CAD build for the part. Positions are in the model's coordinates, mm. Coordinates: 2 decimals unless noted, no trailing zeros. Order: outer loops, then holes, each group sorted by start corner. A loop starts at its lowest first (then second) coordinate and runs counter-clockwise, first axis right, second up.
from build123d import *

# Parameters (mm, degrees)
F1_DEPTH = 25.4


with BuildPart() as f1:
    # F0 (on Front) → F1 (new body)
    with BuildSketch(Plane.XZ):
        with BuildLine():
            Line((44.45, 0), (12.7, 0))
            ThreePointArc((12.7, 0), (8.980256, -8.980256), (0, -12.7))
            Line((0, -12.7), (0, -44.45))
            ThreePointArc((0, -44.45), (4.490128, -46.309872), (6.35, -50.8))
            Line((6.35, -50.8), (12.7, -50.8))
            ThreePointArc((12.7, -50.8), (23.358147, -23.358147), (50.8, -12.7))
            Line((50.8, -12.7), (50.8, -6.35))
            ThreePointArc((50.8, -6.35), (46.309872, -4.490128), (44.45, 0))
        make_face()
        with BuildLine():
            ThreePointArc((0, 12.7), (8.980256, 8.980256), (12.7, 0))
            Line((12.7, 0), (44.45, 0))
            ThreePointArc((44.45, 0), (46.309872, 4.490128), (50.8, 6.35))
            Line((50.8, 6.35), (50.8, 12.7))
            ThreePointArc((50.8, 12.7), (23.358147, 23.358147), (12.7, 50.8))
            Line((12.7, 50.8), (6.35, 50.8))
            ThreePointArc((6.35, 50.8), (4.490128, 46.309872), (0, 44.45))
            Line((0, 44.45), (0, 12.7))
        make_face()
        with BuildLine():
            ThreePointArc((-12.7, 0), (-8.980256, 8.980256), (0, 12.7))
            Line((0, 12.7), (0, 44.45))
            ThreePointArc((0, 44.45), (-4.490128, 46.309872), (-6.35, 50.8))
            Line((-6.35, 50.8), (-12.7, 50.8))
            ThreePointArc((-12.7, 50.8), (-23.358147, 23.358147), (-50.8, 12.7))
            Line((-50.8, 12.7), (-50.8, 6.35))
            ThreePointArc((-50.8, 6.35), (-46.309872, 4.490128), (-44.45, 0))
            Line((-44.45, 0), (-12.7, 0))
        make_face()
        with BuildLine():
            Line((0, -44.45), (0, -12.7))
            ThreePointArc((0, -12.7), (-8.980256, -8.980256), (-12.7, 0))
            Line((-12.7, 0), (-44.45, 0))
            ThreePointArc((-44.45, 0), (-46.309872, -4.490128), (-50.8, -6.35))
            Line((-50.8, -6.35), (-50.8, -12.7))
            ThreePointArc((-50.8, -12.7), (-23.358147, -23.358147), (-12.7, -50.8))
            Line((-12.7, -50.8), (-6.35, -50.8))
            ThreePointArc((-6.35, -50.8), (-4.490128, -46.309872), (0, -44.45))
        make_face()
        with BuildLine():
            Line((50.8, 12.7), (50.8, 6.35))
            ThreePointArc((50.8, 6.35), (55.290128, 4.490128), (57.15, 0))
            ThreePointArc((57.15, 0), (55.290128, -4.490128), (50.8, -6.35))
            Line((50.8, -6.35), (50.8, -12.7))
            ThreePointArc((50.8, -12.7), (63.5, 0), (50.8, 12.7))
        make_face()
        with BuildLine():
            Line((-12.7, 50.8), (-6.35, 50.8))
            ThreePointArc((-6.35, 50.8), (0, 57.15), (6.35, 50.8))
            Line((6.35, 50.8), (12.7, 50.8))
            ThreePointArc((12.7, 50.8), (0, 63.5), (-12.7, 50.8))
        make_face()
        with BuildLine():
            Line((12.7, -50.8), (6.35, -50.8))
            ThreePointArc((6.35, -50.8), (0, -57.15), (-6.35, -50.8))
            Line((-6.35, -50.8), (-12.7, -50.8))
            ThreePointArc((-12.7, -50.8), (0, -63.5), (12.7, -50.8))
        make_face()
        with BuildLine():
            ThreePointArc((-50.8, -6.35), (-57.15, 0), (-50.8, 6.35))
            Line((-50.8, 6.35), (-50.8, 12.7))
            ThreePointArc((-50.8, 12.7), (-63.5, 0), (-50.8, -12.7))
            Line((-50.8, -12.7), (-50.8, -6.35))
        make_face()
    extrude(amount=F1_DEPTH)


solid = f1.part
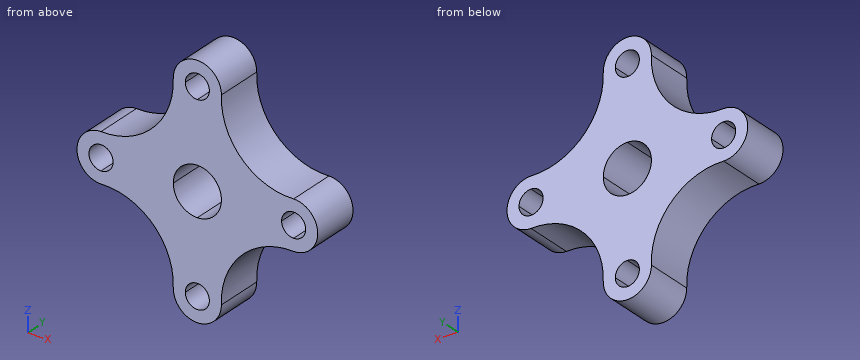
1) Slice it at B-B (z = -54). List the corners of the cut face in (x, y), plus the area to 3 significant figures.
2) Drill centre lines: probe 1 along X at (y, z) = (-23.75, 2); probe 2 along Z at (x, y) = (3.5, -7.5); probe 3 along Z at (x, y) = (49.5, -16.5). Where is each one in solid material? Low to high.
3) Slice it at A-A (y = -6). Give the number of separate pieces and of enclosed holes in the cut face, plus the area to 3 significant figures.
4) Pin check, flat tips, straight feed: P1, Ø2, axis at y = -6.5, z = 2, coming from the -X side; P2, Ø2, axis at x = -48.5, y = -10, coming from the -Z side; P3, Ø10, axis at x = 23.5, y = -8, coming from the +Z side. Stop position of each tip, or through.
5) Slice it at C-C (x = -15). List the corners of the cut face in (y, z).
6) Slice it at D-D (z = 42.5). List the corners of the cut face in (x, y), plus the area to 3 significant figures.
Worked out:
1. outline: (-12.29, -25.4) - (-5.48, -25.4) - (-5.48, 0) - (-12.29, 0) - close; (5.48, -25.4) - (12.29, -25.4) - (12.29, 0) - (5.48, 0) - close
1. area: 346 mm2
2. probe 1: x = -63.34 to -56.83, -44.77 to -12.54, 12.54 to 44.77, 56.83 to 63.34
2. probe 2: z = -63.01 to -56.1, -45.5 to -12.21, 12.21 to 45.5, 56.1 to 63.01
2. probe 3: z = -12.67 to -6.22, 6.22 to 12.67
3. separate pieces: 1
3. enclosed holes: 5
3. area: 5,650 mm2
4. P1: stops at x = -63.46
4. P2: stops at z = -12.7
4. P3: stops at z = 29.37
5. outline: (-25.4, -36.33) - (0, -36.33) - (0, 36.33) - (-25.4, 36.33) - close
6. outline: (-13.28, -25.4) - (13.28, -25.4) - (13.28, 0) - (-13.28, 0) - close
6. area: 675 mm2
